The listing builds one solid part. Answer for the finished solid, in the listing's coordinates (mm). A direction names the side the tool comes from. Give positions to 0.01 mm unless a question says otherwise; leave off trailing zeros. Write each loop counter-clockwise with the first axis right and the second up, starting at its lowest first coordinate (ties: lowest second). Pieces come first, ordered by that corner, then holes. Notation, with made-up numbers: M -36.5,30.25 L -3.5,30.25 A21 cw -3.5,54.25 Z; hole C 34.5,-10.75 d7. An arc over 180 degrees is marked long. Return JSON: item names as keys, results as strings.
from build123d import *

# Parameters (mm, degrees)
SKETCH_W          = 35
SKETCH_H          = 10
PAD_DEPTH         = 7.5
FILLET_R          = 3
SKETCH002_W       = 4
SKETCH002_H       = 28
PAD001_DEPTH      = 4.5
PAD001_DEPTH_BACK = 7.5
FILLET001_R       = 2
SKETCH003_R       = 1.625
SKETCH003_R_2     = 2
POCKET_DEPTH      = 19.501
FILLET002_R       = 4


with BuildPart() as part:
    # Sketch → Pad (new body)
    with BuildSketch(Plane.XY):
        Rectangle(SKETCH_W, SKETCH_H)
        with BuildLine():
            ThreePointArc((-13.5, 1.625), (-15.125, 0), (-13.5, -1.625))
            Line((-13.5, -1.625), (-4.5, -1.625))
            ThreePointArc((-4.5, -1.625), (-2.875, 0), (-4.5, 1.625))
            Line((-13.5, 1.625), (-4.5, 1.625))
        make_face(mode=Mode.SUBTRACT)
        with BuildLine():
            ThreePointArc((4.5, 1.625), (2.875, 0), (4.5, -1.625))
            Line((4.5, -1.625), (13.5, -1.625))
            ThreePointArc((13.5, -1.625), (15.125, 0), (13.5, 1.625))
            Line((4.5, 1.625), (13.5, 1.625))
        make_face(mode=Mode.SUBTRACT)
    extrude(amount=PAD_DEPTH)

    # Fillet
    fillet_edges = [part.edges().sort_by_distance(p)[0] for p in [
        (-17.5, 5, 3.75),
        (-17.5, -5, 3.75),
        (17.5, -5, 3.75),
        (17.5, 5, 3.75),
    ]]
    fillet(fillet_edges, radius=FILLET_R)

    # Sketch002 (on Face5 of Fillet) → Pad001 (join, two sides)
    with BuildSketch(Plane.XY.offset(7.5)) as pad001_sk:
        with Locations((0, 19)):
            Rectangle(SKETCH002_W, SKETCH002_H)
    extrude(amount=PAD001_DEPTH)
    extrude(pad001_sk.sketch, amount=-PAD001_DEPTH_BACK)

    # Fillet001
    fillet001_edges = [part.edges().sort_by_distance(p)[0] for p in [
        (2, 5, 3.75),
        (-2, 5, 3.75),
    ]]
    fillet(fillet001_edges, radius=FILLET001_R)

    # Sketch003 (on Face22 of Fillet001) → Pocket (cut, through all)
    with BuildSketch(Plane(origin=(-2, 0, 0), x_dir=(0, -1, 0), z_dir=(-1, 0, 0))):
        with Locations((-29, 6)):
            Circle(SKETCH003_R)
        with Locations((-11, 6)):
            Circle(SKETCH003_R)
        with Locations((-20, 6)):
            Circle(SKETCH003_R_2)
    extrude(amount=-POCKET_DEPTH, mode=Mode.SUBTRACT)

    # Fillet002
    fillet002_edges = [part.edges().sort_by_distance(p)[0] for p in [
        (0, 33, 0),
        (0, 33, 12),
        (0, 5, 12),
    ]]
    fillet(fillet002_edges, radius=FILLET002_R)


solid = part.part
Item 1: A cutting plane is placed at B-B, the plane y = 11. Write down the section's boundary in (x, z) (3 decimals).
Geometry results:
{"outline": "M -2,0 L 2,0 L 2,4.375 L -2,4.375 Z; M -2,7.625 L 2,7.625 L 2,12 L -2,12 Z"}
Item 2: Given pin 1 Ø1.9 at (y, z) = (29, 6) entering from -X; pin 2 Ø2 at (x, z) = (7, 4.5) entering from +Y; pin 3 Ø1.5 at (y, z) = (3, 8) entering from -X; pin 4 Ø1.5 at (y, z) = (5, 4) entering from +X, each flat-ended and moving along its own axis, determine where each tip first touches the part or whether it passes through.
Geometry results:
{"pin 1": "passes through", "pin 2": "stops at y = 5", "pin 3": "stops at x = -17.47", "pin 4": "stops at x = 16.48"}
Item 3: A cutting plane is placed at C-C, the plane x = 10. Write down the section's boundary in (y, z) (3 decimals), plus the area to 3 significant figures.
Geometry results:
{"outline": "M -5,0 L -1.625,0 L -1.625,7.5 L -5,7.5 Z; M 1.625,0 L 5,0 L 5,7.5 L 1.625,7.5 Z", "area": "50.6 mm2"}
Item 4: A cutting plane is placed at D-D, the plane x = 0.5. Write down the section's boundary in (y, z) (3 decimals).
Geometry results:
{"outline": "M -5,0 L 29,0 A4 ccw 33,4 L 33,8 A4 ccw 29,12 L 9,12 A4 ccw 5,8 L 5,7.5 L -5,7.5 Z; hole C 11,6 d3.25; hole C 20,6 d4; hole C 29,6 d3.25"}
Item 5: Find the intervals of material crossed by line 1 (Y direction, x = -9.5, z = 2.75) (3 decimals); line 2 (Z direction, x = -0.25, y = 20); line 3 (Z direction, x = -0.4, y = 11) (3 decimals), in increasing order.
Geometry results:
{"line 1": "y = -5 to -1.625, 1.625 to 5", "line 2": "z = 0 to 4, 8 to 12", "line 3": "z = 0 to 4.375, 7.625 to 12"}
Item 6: Determine the mould class of faces 4 (the flat face through (-9, -1.625, 4)), 5 (the flat face through (17.5, 0, 4)), 6 (the cylindrical face through (0.028, 31.859, 10.797)), 7 (the flat face through (9, 1.625, 4)) for opening direction X: +X half, -X half, draft (parallel to the pull), parting line (faces both ways), or undercut.
Geometry results:
{"face 4": "undercut", "face 5": "+X half", "face 6": "draft", "face 7": "undercut"}
Item 7: A cutting plane is placed at A-A, the plane z = 6. Count the separate pieces of the cut face and the enclosed holes in it, plus the area to 3 significant figures.
Geometry results:
{"separate pieces": "4", "enclosed holes": "2", "area": "339 mm2"}
Item 8: Which of the six approach directions +Z, -Z, +X, -X, +Y, -Y give full straight-line access (tool end or side, diameter ignored) to faces 1 (the flat face through (-9, 5, 4)), 2 (the flat face through (-17.5, 0, 4)), 3 (the cylindrical face through (15.125, -0.036, 3.698))?
Geometry results:
{"face 1": "+Z, -Z, -X, +Y", "face 2": "+Z, -Z, -X, +Y, -Y", "face 3": "+Z, -Z"}
